Check sheet for the drawn part. Datum: minimum x, y, z corner. Units: mm. Round coordinates to 2 decimals unless told otherwise and drop trailing zeros. Loops run counter-clockwise (first coordinate to the right, second up) from the corner with the lowest first, then second, coordinate; pieces in that order, holes last. Notation, with made-up numbers: (17, 89.5) -> (33, 89.5) arc R20 ccw to (33, 114.5) -> close; hole circle Ø11 at (43.25, 49.25). An arc over 180 degrees is marked (long way). Write item = value, one per line. Start each with the question number.
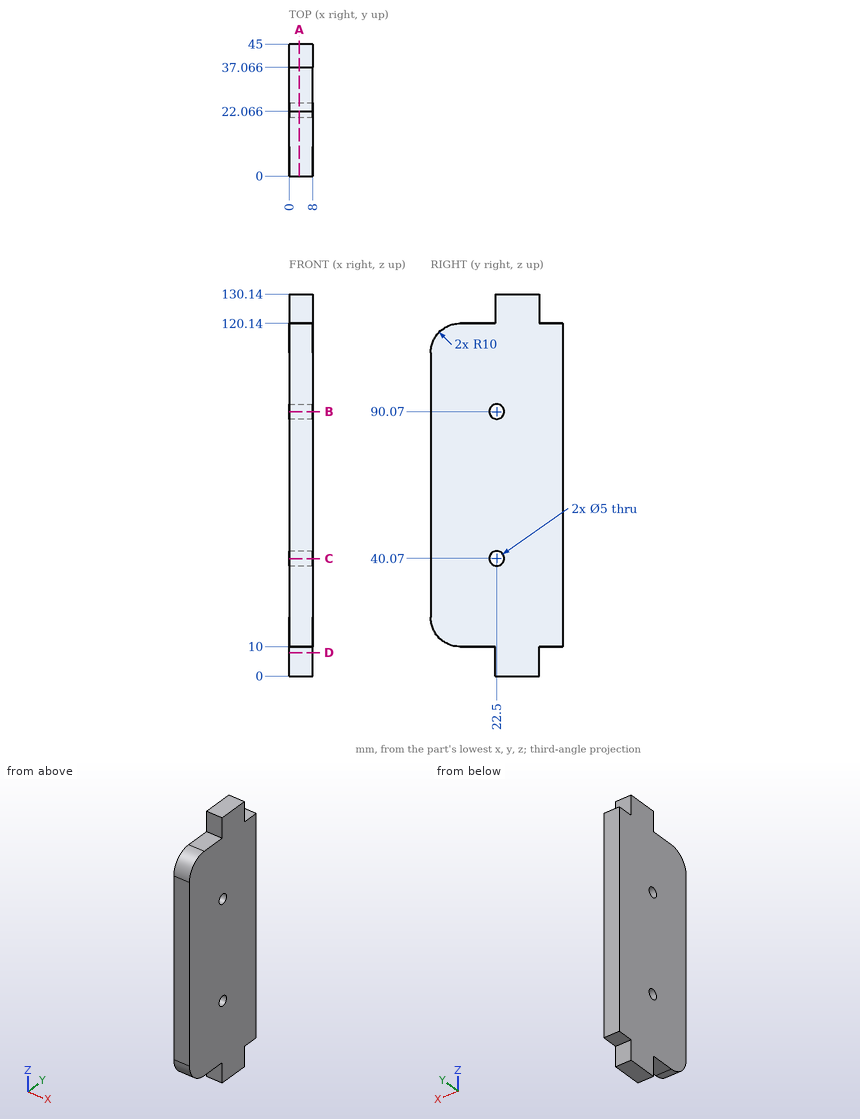
(1) Scan lines: line 1 (Y direction, x = 4.5, z = 40.07); line 2 (Z direction, x = 4.5, y = 21); line 3 (Z direction, x = 4.75, y = 9.5). Record each from-to range of solid material in increasing order. Write a range as [from, to].
(2) Section check D-D on z = 8. Enter the section's corners in (x, y) (1 decimal).
(3) Section check A-A on x = 3.5. Enter the section's corners in (y, z) (1 decimal).
(4) Section check B-B on z = 90.07. Enter the section's corners in (x, y), then the cut area to 3 significant figures.
(5) Depth check by flat-ended pin: pin 1 Ø2.5 at (x, y) = (3, 14) entering from -Z; pin 2 Ø2.5 at (x, z) = (5, 6) entering from +Y; pin 3 Ø2.5 at (x, z) = (4.5, 125.5) entering from -Y. Enter the tip coordinate at first touch or a pass-through.
Computed values:
q1.line_1 = [0, 20], [25, 45]
q1.line_2 = [10, 38.07], [42.07, 88.07], [92.07, 120.14]
q1.line_3 = [10.01, 120.13]
q2.outline = (0, 22.1) -> (8, 22.1) -> (8, 37.1) -> (0, 37.1) -> close
q3.outline = (0, 20) arc R10 ccw to (10, 10) -> (22.1, 10) -> (22.1, 0) -> (37.1, 0) -> (37.1, 10) -> (45, 10) -> (45, 120.1) -> (37.1, 120.1) -> (37.1, 130.1) -> (22.1, 130.1) -> (22.1, 120.1) -> (10, 120.1) arc R10 ccw to (0, 110.1) -> close; hole circle Ø5 at (22.5, 40.1); hole circle Ø5 at (22.5, 90.1)
q4.outline = (0, 0) -> (8, 0) -> (8, 20) -> (0, 20) -> close; (0, 25) -> (8, 25) -> (8, 45) -> (0, 45) -> close
q4.area = 320 mm²
q5.pin_1 = 10
q5.pin_2 = 37.07
q5.pin_3 = 22.07
